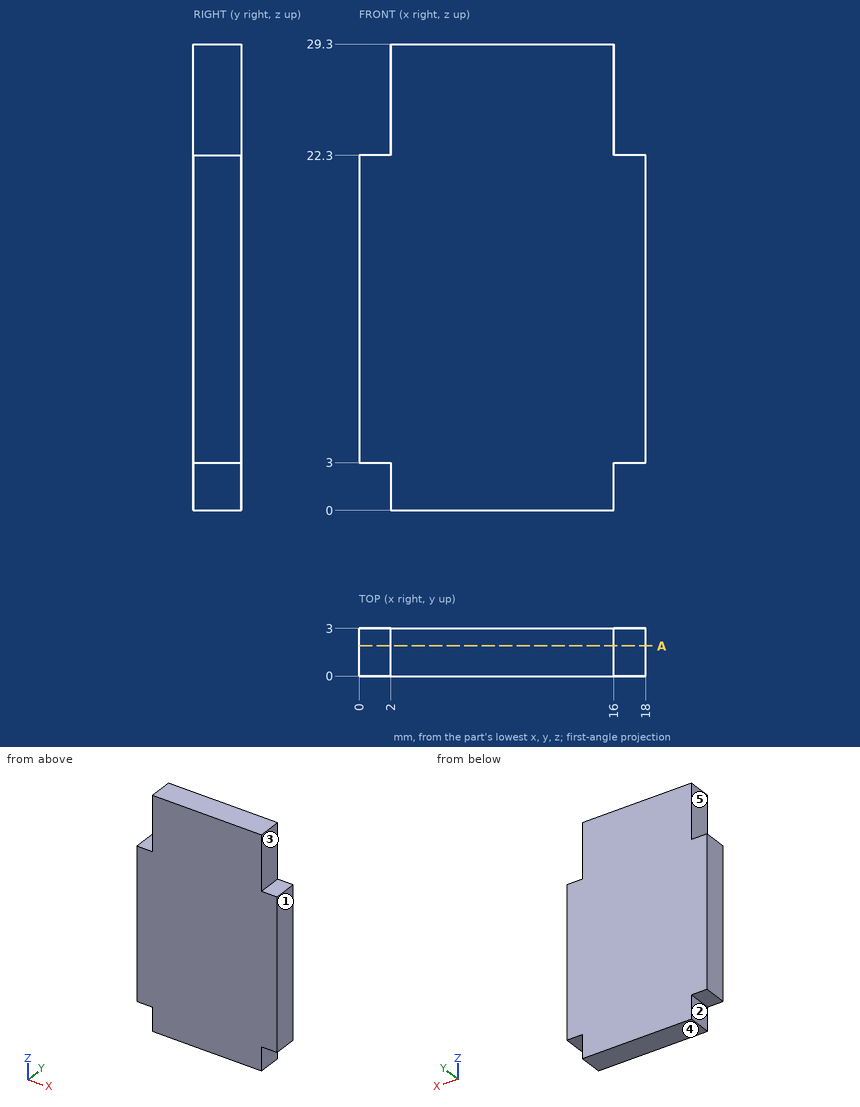
Answer from the drawing. Dimensions are ordinates in mm from the lowest x, y and z of the part. A direction names the side the tool comes from. Round coordinates to 2 decimals unless told otherwise and drop trailing zeros. Order: outer loops, then holes, each group sorted by start corner. A loop starts at its lowest first (then second) coordinate and runs counter-clockwise, first axis right, second up.
1) For the marked faces 1, 2, 3, 4 and 5, determine the directions among +Z, -Z, +X, -X, +Y, -Y from which every point of the face is accessible in a straight line to the end or side of a thin tool.
2) The part is cut by section A-A on y = 1.9. Write down the section's boundary in (x, z), plus the area to 3 significant figures.
3) A straight line is drawn through the part: L1, parallel to X at y = 2.3, z = 25.25. Find the intervals that lie inside material, in ascending order.
4) Flat-ended cylindrical pins translate along their axes: pin 1 (1 mm diameter, centred on x = 1, y = 1, fed in from +Z); pin 2 (1.5 mm diameter, centred on y = 1, z = 1.5, fed in from +X). Find the tip coordinate at first contact, or state that the pin passes through.
Resolved:
1. face 1: +Z, -Z, +X, +Y, -Y
1. face 2: -Z, -X, +Y, -Y
1. face 3: +Z, +X, +Y, -Y
1. face 4: -Z, +X, -X, +Y, -Y
1. face 5: +Z, -X, +Y, -Y
2. outline: (0, 3) - (2, 3) - (2, 0) - (16, 0) - (16, 3) - (18, 3) - (18, 22.3) - (16, 22.3) - (16, 29.3) - (2, 29.3) - (2, 22.3) - (0, 22.3) - close
2. area: 487 mm2
3. L1: x = 2 to 16
4. pin 1: stops at z = 22.3
4. pin 2: stops at x = 16
